Work out the finished part from the listing and answer in its coordinate system (mm). Coordinates: 2 decimals unless noted, no trailing zeros. Write each loop counter-clockwise with the first axis right and the second up, starting at its lowest first coordinate (ties: lowest second). Pieces come first, ordered by that corner, then holes. Notation, with made-up numbers: (79, 36) - (89, 36) arc R8 cw to (89, 42) - close; hole circle Ø2 at (41, 45.5). An arc over 180 degrees is marked (long way). Use CSV: the item, a comma, the result in double quotes. Start each with the question number.
from build123d import *

# Parameters (mm, degrees)
SKETCH1_W                   = 60
SKETCH1_H                   = 16.957284299
BOSS_EXTRUDE1_DEPTH         = 5
TAP_DRILL_FOR_M2X0_4_TAP1_D = 1.6


with BuildPart() as part:
    # Sketch1 → Boss-Extrude1 (new body)
    with BuildSketch(Plane(origin=(0, 0, 0), x_dir=(1, 0, 0), z_dir=(0, 1, 0))):
        with Locations((-20.230276441, -316.427173265)):
            Rectangle(SKETCH1_W, SKETCH1_H)
    extrude(amount=BOSS_EXTRUDE1_DEPTH)

    # Tap Drill for M2x0.4 Tap1 (through all)
    with Locations(Plane.XY.offset(324.905815414)):
        with Locations((-44.406835203, 2.5)):
            Hole(TAP_DRILL_FOR_M2X0_4_TAP1_D / 2)


solid = part.part
Item 1: Determine the mould class of faces 1 (the face through (-21, 2, 324.906)), 2 (the face through (-43.608, 2.535, 316.308)), 3 (the face through (-21, 5, 316)) for opening direction Y: +Y half, -Y half, draft (parallel to the pull), parting line (faces both ways), or undercut.
Item 2: A cutting plane is placed at A-A (y = 2.5). Determine the outline of the cut face in (x, z), then the cut area to 3 significant figures.
Item 3: Straight lines are drawn through the part: probe 1 along X at (y, z) = (1.85, 318); probe 2 along X at (y, z) = (2.75, 312.75). For each, find the intervals that lie inside material, in ascending order. Write a range as [from, to].
Calculated:
1,face 1,"draft"
1,face 2,"undercut"
1,face 3,"+Y half"
2,outline,"(-50.23, 307.95) - (-45.21, 307.95) - (-45.21, 324.91) - (-50.23, 324.91) - close; (-43.61, 307.95) - (9.77, 307.95) - (9.77, 324.91) - (-43.61, 324.91) - close"
2,area,"990 mm²"
3,probe 1,"x = [-50.23, -44.87], [-43.94, 9.77]"
3,probe 2,"x = [-50.23, -45.17], [-43.65, 9.77]"
